Source: CAD feature listing. Evaluate the final solid. Frame: model axes, mm. Coordinates: 2 decimals unless noted, no trailing zeros. Order: outer loops, then holes, each group sorted by start corner. A loop starts at its lowest first (then second) coordinate and runs counter-clockwise, first axis right, second up.
```python
from build123d import *

# Parameters (mm, degrees)
ESQUISSE1_W      = 1.5
ESQUISSE1_H      = 1.5
FENTE_REACH      = 10.298
FENTE_END_RADIUS = 2.15


with BuildPart() as part:
    # Esquisse1 → Base (revolve)
    with BuildSketch(Plane.XY, mode=Mode.PRIVATE) as base_sk:
        with Locations((2.9, 0.75)):
            Rectangle(ESQUISSE1_W, ESQUISSE1_H)
    revolve(base_sk.sketch.rotate(Axis((0, 0.5, 0), (0, -1, 0)), 90), axis=Axis((0, 0.5, 0), (0, -1, 0)))

    # Fente: up to this cylinder (the profile starts outside it)
    fente_end = Plane(origin=(0, 0.75, 0), z_dir=(0, 1, 0)) * Cylinder(FENTE_END_RADIUS, 25.896, mode=Mode.PRIVATE)
    # Esquisse2 → Fente (cut, up to the surface)
    with BuildSketch(Plane.XY.offset(3.65), mode=Mode.PRIVATE) as fente_sk1:
        Polygon((-0.474368226, 2.230588572), (-0.072444437, 0.730588572), (0.329479352, -0.769411428), (0.474368226, -0.730588572), (0.072444437, 0.769411428), (-0.329479352, 2.269411428), align=None)
    fente_tool1 = extrude(fente_sk1.sketch, amount=-FENTE_REACH, mode=Mode.PRIVATE) - fente_end
    add(fente_tool1.solids().sort_by_distance((0, 0.75, 3.65))[0], mode=Mode.SUBTRACT)


solid = part.part
```
Q1. Pull-direction query (Y, two-part tool) for faces 1 (the flat face through (-0.036, 0.594, 2.902)), 2 (the flat face through (2, 1.5, -2)), 3 (the flat face through (2, 0, -2)); classes: pulls with the +Y half, pulls with the -Y half, needs draft (parallel to the pull), parting line crosses it, or undercut.
Solutions:
face 1: undercut
face 2: pulls with the +Y half
face 3: pulls with the -Y half
Q2. Section query C-C on y = 1.3. Output: boundary loops of the cut face in (x, z).
Solutions:
outline: (-0.23, 2.14) - (-0.23, 3.64) arc R3.65 ccw (long way) to (-0.07, 3.65) - (-0.07, 2.15) arc R2.15 cw (long way) to start
Q3. Section query B-B on x = 2. Output: boundary loops of the cut face in (y, z), plus the area to 3 significant figures.
Solutions:
outline: (0, -3.05) - (1.5, -3.05) - (1.5, -0.79) - (0, -0.79) - close; (0, 0.79) - (1.5, 0.79) - (1.5, 3.05) - (0, 3.05) - close
area: 6.79 mm2
Q4. Material intervals for line 1 along X through (y, z) = (0.35, 0); line 2 along Z through (x, y) = (0.75, 0.95); line 3 along Z through (x, y) = (0, 0.9), sorted ascending.
Solutions:
line 1: x = -3.65 to -2.15, 2.15 to 3.65
line 2: z = -3.57 to -2.01, 2.01 to 3.57
line 3: z = -3.65 to -2.15
Q5. Section query A-A on z = 0. Output: boundary loops of the cut face in (x, y).
Solutions:
outline: (-3.65, 0) - (-2.15, 0) - (-2.15, 1.5) - (-3.65, 1.5) - close; (2.15, 0) - (3.65, 0) - (3.65, 1.5) - (2.15, 1.5) - close
Q6. Section query D-D on x = -2.75. Output: boundary loops of the cut face in (y, z), plus the area to 3 significant figures.
Solutions:
outline: (0, -2.4) - (1.5, -2.4) - (1.5, 2.4) - (0, 2.4) - close
area: 7.20 mm2
